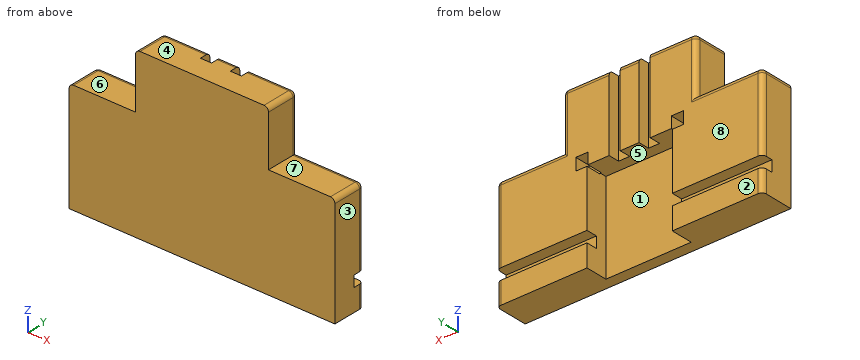
```python
from build123d import *

# Parameters (mm, degrees)
SKETCH1_W                                  = 120
SKETCH1_H                                  = 100
BOSS_EXTRUDE1_DEPTH                        = 15
SKETCH7_W                                  = 60
SKETCH7_H                                  = 25
BOSS_EXTRUDE6_DEPTH                        = 15
FILLET1_R                                  = 2
SKETCH2_W                                  = 38.5
SKETCH2_H                                  = 82
CUT_EXTRUDE1_DEPTH                         = 10
CUT_EXTRUDE3_DEPTH                         = 5
SKETCH11_W                                 = 5.5
SKETCH11_H                                 = 5.5
CUT_EXTRUDE6_DEPTH                         = 7
MIRROR3_AT_THE_SECOND_PLANE_COPY_1_SKETC_W = 5.5
MIRROR3_AT_THE_SECOND_PLANE_COPY_1_SKETC_H = 5.5
MIRROR3_AT_THE_SECOND_PLANE_COPY_1_DEPTH   = 7
MIRROR4_AT_THE_SECOND_PLANE_COPY_1_DEPTH   = 5
CUT_EXTRUDE7_REACH                         = 99.211
SKETCH12_W                                 = 131.778064034
SKETCH12_H                                 = 21.740712993


with BuildPart() as part:
    # Sketch1 → Boss-Extrude1 (new body)
    with BuildSketch(Plane(origin=(0, 0, 0), x_dir=(1, 0, 0), z_dir=(0, 1, 0))):
        Rectangle(SKETCH1_W, SKETCH1_H)
    extrude(amount=BOSS_EXTRUDE1_DEPTH)

    # Sketch7 → Boss-Extrude6 (add)
    with BuildSketch(Plane(origin=(0, 0, 0), x_dir=(1, 0, 0), z_dir=(0, 1, 0))):
        with Locations((0, -62.5)):
            Rectangle(SKETCH7_W, SKETCH7_H)
        with Locations((0, 62.5)):
            Rectangle(SKETCH7_W, SKETCH7_H)
    extrude(amount=BOSS_EXTRUDE6_DEPTH)

    # Fillet1
    fillet1_edges = [part.edges().sort_by_distance(p)[0] for p in [
        (-60, 15, 0),
        (45, 15, 50),
        (-45, 15, 50),
        (-30, 7.5, 75),
        (30, 7.5, 75),
        (-30, 15, 62.5),
        (0, 15, 75),
        (30, 15, 62.5),
        (-45, 15, -50),
        (0, 15, -75),
        (30, 7.5, -75),
        (-30, 15, -62.5),
        (-30, 7.5, -75),
        (30, 15, -62.5),
        (60, 15, 0),
        (60, 7.5, 50),
        (-60, 7.5, 50),
        (-60, 7.5, -50),
        (60, 7.5, -50),
        (45, 15, -50),
    ]]
    fillet(fillet1_edges, radius=FILLET1_R)

    # Sketch2 → Cut-Extrude1 (cut)
    with BuildSketch(Plane(origin=(0, 15, 0), x_dir=(1, 0, 0), z_dir=(0, 1, 0))):
        Rectangle(SKETCH2_W, SKETCH2_H)
    extrude(amount=-CUT_EXTRUDE1_DEPTH, mode=Mode.SUBTRACT)

    # Sketch10 → Cut-Extrude3 (cut)
    with BuildSketch(Plane(origin=(0, 15, 0), x_dir=(1, 0, 0), z_dir=(0, 1, 0))):
        Polygon((-9.25, -40.5), (-9.25, -33.162899401), (-4.25, -33.162899401), (-4.25, -40.5), (-4.25, -89.766264028), (-9.25, -89.766264028), align=None)
        Polygon((-82.808425803, 15), (-19.25, 15), (-11.555108838, 15), (-11.555108838, 10), (-19.25, 10), (-82.808425803, 10), align=None)
    cut_extrude3 = extrude(amount=-CUT_EXTRUDE3_DEPTH, mode=Mode.SUBTRACT)

    # Sketch11 → Cut-Extrude6 (cut)
    with BuildSketch(Plane(origin=(0, 15, 0), x_dir=(1, 0, 0), z_dir=(0, 1, 0))):
        with Locations((-21.549732367, 43.299732367)):
            Rectangle(SKETCH11_W, SKETCH11_H)
    cut_extrude6 = extrude(amount=-CUT_EXTRUDE6_DEPTH, mode=Mode.SUBTRACT)

    # Mirror3: Cut-Extrude6 across plane
    add(cut_extrude6.mirror(Plane(origin=(0, 0, 0), x_dir=(0, 0, 1), z_dir=(1, 0, 0))), mode=Mode.SUBTRACT)

    # Mirror3 at the second plane: Cut-Extrude6 across plane
    add(cut_extrude6.mirror(Plane.XY), mode=Mode.SUBTRACT)

    # Mirror3 at the second plane copy 1 sketc → Mirror3 at the second plane copy 1 (cut)
    with BuildSketch(Plane(origin=(0, 15, 0), x_dir=(-1, 0, 0), z_dir=(0, 1, 0))):
        with Locations((-21.549732367, 43.299732367)):
            Rectangle(MIRROR3_AT_THE_SECOND_PLANE_COPY_1_SKETC_W, MIRROR3_AT_THE_SECOND_PLANE_COPY_1_SKETC_H)
    extrude(amount=-MIRROR3_AT_THE_SECOND_PLANE_COPY_1_DEPTH, mode=Mode.SUBTRACT)

    # Mirror4: Cut-Extrude3 across plane
    add(cut_extrude3.mirror(Plane(origin=(0, 0, 0), x_dir=(0, 0, 1), z_dir=(1, 0, 0))), mode=Mode.SUBTRACT)

    # Mirror4 at the second plane: Cut-Extrude3 across plane
    add(cut_extrude3.mirror(Plane.XY), mode=Mode.SUBTRACT)

    # Mirror4 at the second plane copy 1 sketc → Mirror4 at the second plane copy 1 (cut)
    with BuildSketch(Plane(origin=(0, 15, 0), x_dir=(-1, 0, 0), z_dir=(0, 1, 0))):
        Polygon((-9.25, -40.5), (-9.25, -33.162899401), (-4.25, -33.162899401), (-4.25, -40.5), (-4.25, -89.766264028), (-9.25, -89.766264028), align=None)
        Polygon((-82.808425803, 15), (-19.25, 15), (-11.555108838, 15), (-11.555108838, 10), (-19.25, 10), (-82.808425803, 10), align=None)
    extrude(amount=-MIRROR4_AT_THE_SECOND_PLANE_COPY_1_DEPTH, mode=Mode.SUBTRACT)

    # Sketch12 → Cut-Extrude7 (cut, up to next)
    with BuildSketch(Plane.XY, mode=Mode.PRIVATE) as cut_extrude7_sk1:
        with Locations((-0.266757215, 8.03351443)):
            Rectangle(SKETCH12_W, SKETCH12_H)
    cut_extrude7_tool1 = extrude(cut_extrude7_sk1.sketch, amount=-CUT_EXTRUDE7_REACH, mode=Mode.PRIVATE) & part.part
    add(cut_extrude7_tool1.solids().sort_by_distance((-0.266757, 8.033514, 0))[0], mode=Mode.SUBTRACT)


solid = part.part
```
The model under review builds one solid part; all positions refer to its coordinate system, in mm. Face numbers are marked on the shaded views. A direction names the side the tool comes from. Coordinates: 2 decimals unless noted, no trailing zeros. Order: outer loops, then holes, each group sorted by start corner. A loop starts at its lowest first (then second) coordinate and runs counter-clockwise, first axis right, second up. Notation, with made-up numbers: M 29.5,-11 L 46.5,-11 A21 ccw 46.5,15 Z; hole C -16.5,29 d6. An arc over 180 degrees is marked long. One line per question, with ' | ' between items.
(1) Insertion check: pin 1 (5 mm diameter, centred on x = 39.5, y = 12, fed in from +Z); pin 2 (2.5 mm diameter, centred on x = 7.5, z = 53.5, fed in from +Y); pin 3 (2 mm diameter, centred on x = 6, z = 35, fed in from +Y). Each pin has a flat end and moves straight along its axis. Give the tip position at first contact, or say it passes through.
Geometry results:
pin 1: stops at z = 50 | pin 2: stops at y = 10 | pin 3: stops at y = 5
(2) Add section A-A, the plane y = 3. Write out the cut boundary in (x, z).
Geometry results:
outline: M -60,0 L 60,0 L 60,48 A2 ccw 58,50 L 30,50 L 30,73 A2 ccw 28,75 L -28,75 A2 ccw -30,73 L -30,50 L -58,50 A2 ccw -60,48 Z
(3) The part is to be moulded in two halves that separate along X. For the marked faces 1, 2 and 3, say which applies: +X half, -X half, draft (parallel to the pull), parting line (faces both ways), or undercut.
Geometry results:
face 1: undercut | face 2: draft | face 3: +X half
(4) Add section B-B, the plane x = 2.5. Write out the cut boundary in (y, z).
Geometry results:
outline: M 0,0 L 5,0 L 5,41 L 15,41 L 15,73 A2 ccw 13,75 L 0,75 Z
(5) Add section C-C, the plane z = 30. Write out the cut boundary in (x, y), then the cut area to 3 significant figures.
Geometry results:
outline: M -60,0 L 60,0 L 60,13 A2 ccw 58,15 L 19.25,15 L 19.25,5 L -19.25,5 L -19.25,15 L -58,15 A2 ccw -60,13 Z | area: 1,410 mm²
(6) Machinability: for the marked faces 4, 5, 6, 7 and 8, which of the approach directions +Z, -Z, +X, -X, +Y, -Y give a long, thin tool a straight path to every point of the face, cutting with its end or side? Answer none if there is none.
Geometry results:
face 4: +Z, +X, -X, +Y, -Y | face 5: -Z, +Y | face 6: +Z, -X, +Y, -Y | face 7: +Z, +X, +Y, -Y | face 8: +Z, -Z, +X, -X, +Y
(7) For probe 1 along X at (y, z) = (12.5, 64); probe 2 along X at (y, z) = (7, 26.5); probe 3 along Z at (x, y) = (31.5, 10.5), list the stretches that pass through material, from the lowest coordinate up. Write a range as from..to.
Geometry results:
probe 1: x = -30..-9.25, -4.25..4.25, 9.25..30 | probe 2: x = -60..-19.25, 19.25..60 | probe 3: z = 0..10, 15..50
(8) Add section D-D, the plane y = 11.25. State how many separate pieces and enclosed holes the cut face has, then the cut area to 3 significant figures.
Geometry results:
separate pieces: 5 | enclosed holes: 0 | area: 5,110 mm²
